```python
from build123d import *

# Parameters (mm, degrees)
F0_W     = 25.4
F0_H     = 25.4
F0_R     = 1.778
F1_DEPTH = 10.16
F2_R     = 3.175


with BuildPart() as f1:
    # F0 (on Front) → F1 (new body)
    with BuildSketch(Plane.XZ):
        with Locations((18.961715, -10.547113)):
            Rectangle(F0_W, F0_H)
        with Locations((18.961715, -10.547113)):
            Circle(F0_R, mode=Mode.SUBTRACT)
    extrude(amount=F1_DEPTH)

    # F2
    f2_edges = [f1.edges().sort_by_distance(p)[0] for p in [
        (6.261715, -10.16, -10.547113),
        (31.661715, -10.16, -10.547113),
    ]]
    fillet(f2_edges, radius=F2_R)


solid = f1.part
```
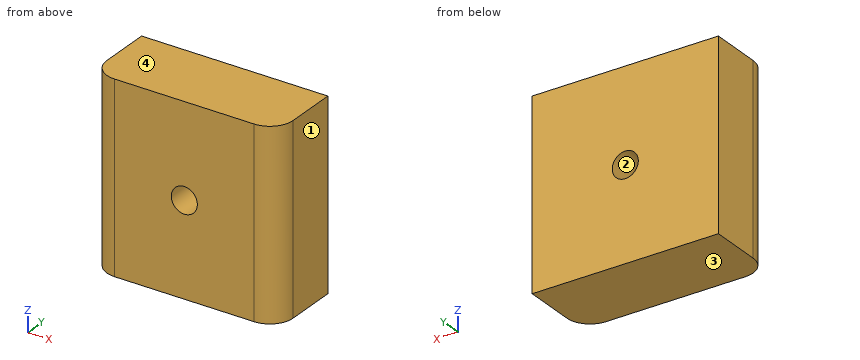
Design review of the part built by this model. Coordinates are the model's own, in mm. Face numbers are marked on the shaded views. Give positions to 0.01 mm unless a question says otherwise; leave off trailing zeros. Order: outer loops, then holes, each group sorted by start corner. A loop starts at its lowest first (then second) coordinate and runs counter-clockwise, first axis right, second up. Notation, with made-up numbers: M 80.5,-26 L 127.5,-26 A34 cw 127.5,8 Z; hole C -27,37 d6. An arc over 180 degrees is marked long. One line per question, with ' | ' between items. Start each with the question number.
Q1. For L1, parallel to Y at x = 9.25, z = -9; L2, parallel to Z at x = 19.5, y = -2.5; L3, parallel to X at y = -8.75, z = -9.25, list the stretches that pass through material, from the lowest coordinate up. Write a range as [from, to].
Q2. For pin 1 Ø3 at (x, z) = (18.96, -10.55) entering from +Y, flat-tipped, find the tip position at first contact; note if it passes through.
Q3. We need section A-A (z = -12.75). Write out the cut boundary in (x, y) (3 decimals), plus the area to 3 significant figures.
Q4. The part is to be moulded in two halves that separate along Z. For the marked faces 1, 2, 3 and 4, say which applies: +Z half, -Z half, draft (parallel to the pull), parting line (faces both ways), or undercut.
Q5. We need section B-B (y = -6.25). Write out the cut boundary in (x, z).
Q6. We need section C-C (x = 29.5). Write out the cut boundary in (y, z), plus the area to 3 significant figures.
Returned:
1) L1: [-10.15, 0] | L2: [-23.25, -12.24], [-8.85, 2.15] | L3: [6.8, 17.75], [20.18, 31.13]
2) pin 1: through
3) outline: M 6.262,-6.985 A3.175 ccw 9.437,-10.16 L 28.487,-10.16 A3.175 ccw 31.662,-6.985 L 31.662,0 L 6.262,0 Z | area: 254 mm2
4) face 1: draft | face 2: undercut | face 3: -Z half | face 4: +Z half
5) outline: M 6.26,-23.25 L 31.66,-23.25 L 31.66,2.15 L 6.26,2.15 Z; hole C 18.96,-10.55 d3.56
6) outline: M -9.99,-23.25 L 0,-23.25 L 0,2.15 L -9.99,2.15 Z | area: 254 mm2
